The drawing under review shows one solid part. Ordinate dimensions are in mm from its lowest x, y, z. A direction names the side the tool comes from. Give positions to 0.01 mm unless a question says otherwise; leave off trailing zeros. Loops run counter-clockwise (first coordinate to the right, second up) from the corner with the lowest first, then second, coordinate; pieces in that order, holes last. Notation, with made-up numbers: M -38,-34.5 L -15,-34.5 A12 ccw -15,-20.5 Z; hole C 28,44 d9. An arc over 180 degrees is marked long. Answer as CSV lines item,"result".
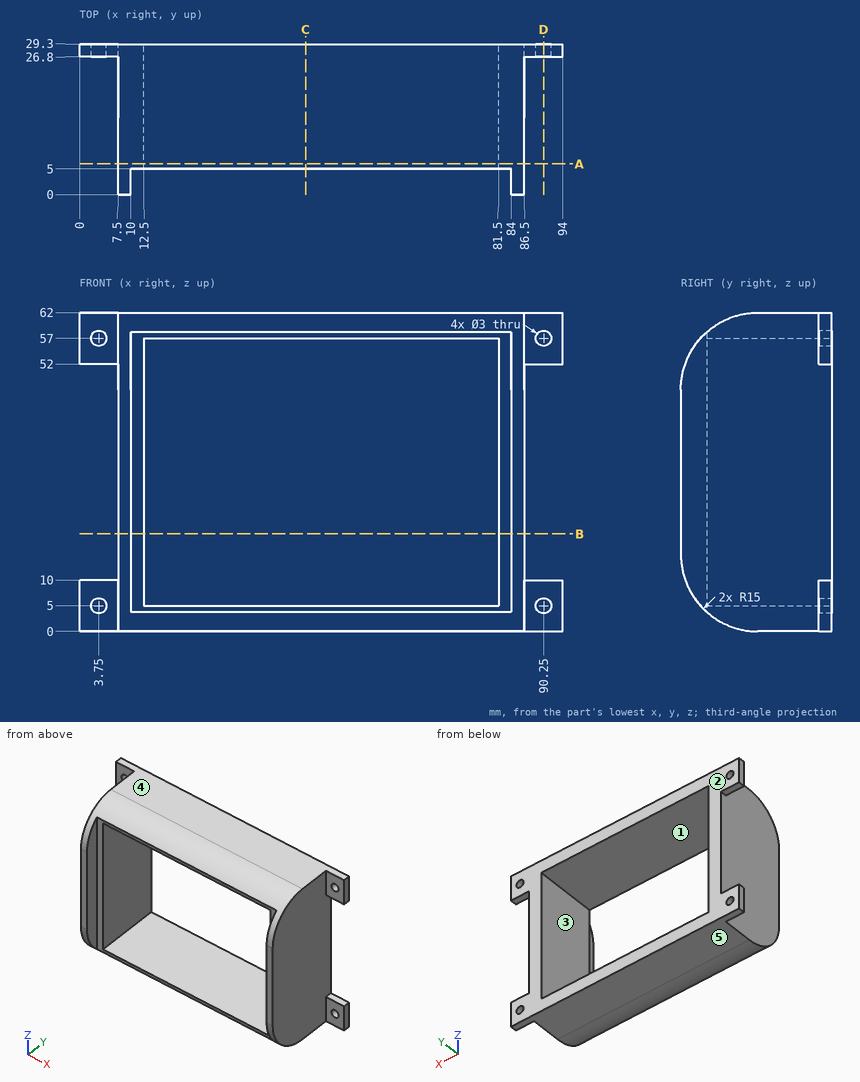
1. We need section B-B, the plane z = 19. Write out the cut boundary in (x, y).
Answer block:
outline,"M 7.5,0 L 10,0 L 10,5 L 12.5,5 L 12.5,29.3 L 7.5,29.3 Z; M 81.5,5 L 84,5 L 84,0 L 86.5,0 L 86.5,29.3 L 81.5,29.3 Z"
2. The part is to be moulded in two halves that separate along Z. For the marked faces 3, 4 and 5, say which applies: pulls with the +Z half, pulls with the -Z half, needs draft (parallel to the pull), parting line crosses it, or undercut.
Answer block:
face 3,"undercut"
face 4,"pulls with the +Z half"
face 5,"pulls with the -Z half"
3. To check wall thickness, follow L1, parallel to Z at x = 90.25, y = 27.85; L2, parallel to X at y = 23, z = 19.5; L3, parallel to Z at x = 40.5, y = 19.25. State the ranges of each line that lie inside material, in increasing order. Write a range as [from, to].
Answer block:
L1,"[0, 3.5], [6.5, 10], [52, 55.5], [58.5, 62]"
L2,"[7.5, 12.5], [81.5, 86.5]"
L3,"[0, 5], [57, 62]"
4. For the marked faces 1 and 2, list the 3-axis set-ups (+Z, -Z, +X, -X, +Y, -Y) from which the entire face can be reached by the end or side of a thin tool; tool diameter is ignored.
Answer block:
face 1,"+Y, -Y"
face 2,"+Z, -Z, +X, -X, +Y"
5. We need section C-C, the plane x = 44. Write out the cut boundary in (y, z), plus the area to 3 significant figures.
Answer block:
outline,"M 5,3.82 A15 ccw 15,0 L 29.3,0 L 29.3,5 L 5,5 Z; M 5,57 L 29.3,57 L 29.3,62 L 15,62 A15 ccw 5,58.18 Z"
area,"219 mm²"
6. We need section D-D, the plane x = 90.25. Write out the cut boundary in (y, z).
Answer block:
outline,"M 26.8,0 L 29.3,0 L 29.3,3.5 L 26.8,3.5 Z; M 26.8,6.5 L 29.3,6.5 L 29.3,10 L 26.8,10 Z; M 26.8,52 L 29.3,52 L 29.3,55.5 L 26.8,55.5 Z; M 26.8,58.5 L 29.3,58.5 L 29.3,62 L 26.8,62 Z"
7. For P1, Ø1.8, axis at x = 90.25, z = 5, coming from the +Y side; P2, Ø10, axis at x = 62, y = 9, coming from the -Z side; P3, Ø9, axis at y = 11, z = 18, coming from the +X side; P4, Ø1.5, axis at y = 3, z = 36, coming from the -X side, all flat-tipped, find the tip position at first contact; note any pin that passes through.
Answer block:
P1,"through"
P2,"z = 0.03"
P3,"x = 86.5"
P4,"x = 7.5"
8. We need section A-A, the plane y = 6. Write out the cut boundary in (x, z), plus the area to 3 significant figures.
Answer block:
outline,"M 7.5,3 L 86.5,3 L 86.5,59 L 7.5,59 Z; hole M 12.5,5 L 81.5,5 L 81.5,57 L 12.5,57 Z"
area,"836 mm²"
